Geometry check sheet. Reference: the model listing, model coordinates, mm. A direction names the side the tool comes from. Round coordinates to 2 decimals unless told otherwise and drop trailing zeros. Write each loop counter-clockwise with the first axis right and the second up, starting at its lowest first coordinate (ties: lowest second). Pieces come first, ordered by that corner, then holes.
Item 1: Cross-section at C-C (y = -19.05). Enter the section's corners in (x, z).
Item 2: Cross-section at B-B (x = 39.37). Enter the section's corners in (y, z).
Item 3: Access from +Z, -Z, +X, -X, +Y, -Y to the whole of each face (thin tool, end or side, straight path). Record for faces 1 (the face through (2, 25.38, 4)), 2 (the face through (42.481, -24, 4)), 3 (the face through (-26.433, -24, 4)).
Item 4: Scan lines: probe 1 along Y at (x, z) = (-3, 3.75); probe 2 along Y at (x, z) = (39.37, -0.65); probe 3 along Y at (x, z) = (-36.83, -1.2). Record each from-to range of solid material in increasing order.
Item 5: Cross-section at A-A (z = 4.25). Enter the section's corners in (x, y).
Item 6: Draft check along Y on faces 4 (the face through (-36.14, -25.46, -0.84)), 5 (the face through (2, 24, 8.34)), 6 (the face through (44, -20.35, 4)). Enter one of: pulls with the +Y half, pulls with the -Y half, needs draft (parallel to the pull), parting line crosses it, or undercut.
Item 7: Depth check by flat-ended pin: P1, Ø1, axis at x = -15, z = 1.5, coming from the -Y side; P2, Ø1.9, axis at y = 20, z = -0.5, coming from the +X side; P3, Ø3, axis at y = -24.5, z = 4, coming from the -X side; P4, Ø5, axis at x = 14, z = 1.5, coming from the -Y side. Enter the tip coordinate at first touch or a pass-through.
Item 8: Cross-section at D-D (y = -9). Enter the section's corners in (x, z), then the cut area to 3 significant figures.
Autodesk Fusion 360 part; units mm, degrees
sketch "Boceto1" plane through (0, 0, 0) normal (0, 0, 1) x (1, 0, 0)
  line L0 (-50.8, 26.67) -> (50.8, 26.67)
  line L1 (50.8, 26.67) -> (50.8, -26.67)
  line L2 (50.8, -26.67) -> (-50.8, -26.67)
  line L3 (-50.8, -26.67) -> (-50.8, 26.67)
  line L4 (-50.8, 0) -> (50.8, 0) construction
  circle A0 centre (-35.56, 24.13) radius 1.5
  circle A1 centre (39.37, 24.13) radius 1.5
  circle A2 centre (45.72, -24.13) radius 1.5
  circle A3 centre (-36.83, -24.13) radius 1.5
  circle A4 centre (15.24, -19.05) radius 1.5
  line L5 (45.2477, 26.67) -> (47.6517, 24.3349)
  line L6 (47.6517, 24.3349) -> (47.6517, 13.9338)
  line L7 (47.6517, 13.9338) -> (50.8, 10.0089)
  line L8 (47.6442, -26.67) -> (47.6442, -25.5537)
  line L9 (47.6442, -25.5537) -> (50.8, -23.002)
  line L10 (-32.1884, 25.38) -> (36.3857, 25.38)
  line L11 (36.3857, 25.38) -> (36.3857, 22.88)
  line L12 (36.3857, 22.88) -> (-32.1884, 22.88)
  line L13 (-32.1884, 22.88) -> (-32.1884, 25.38)
  line L14 (-32.1884, 25.38) -> (36.3857, 22.88) construction
  line L15 (36.3857, 25.38) -> (-32.1884, 22.88) construction
  line L16 (43.14, 24.13) -> (45.64, 24.13)
  line L17 (45.64, 24.13) -> (45.64, -20.35)
  line L18 (45.64, -20.35) -> (43.14, -20.35)
  line L19 (43.14, -20.35) -> (43.14, 24.13)
  line L20 (43.14, 24.13) -> (45.64, -20.35) construction
  line L21 (45.64, 24.13) -> (43.14, -20.35) construction
  line L22 (-26.4326, -22.88) -> (42.4806, -22.88)
  line L23 (42.4806, -22.88) -> (42.4806, -25.38)
  line L24 (42.4806, -25.38) -> (-26.4326, -25.38)
  line L25 (-26.4326, -25.38) -> (-26.4326, -22.88)
  line L26 (-26.4326, -22.88) -> (42.4806, -25.38) construction
  line L27 (42.4806, -22.88) -> (-26.4326, -25.38) construction
  point P0 (2.0986, 24.13)
  point P1 (44.39, 1.89)
  point P2 (8.024, -24.13)
  dimension "d2" = 53.34
  dimension "d3" = 101.6
  dimension "d4" = 13.97
  dimension "d5" = 15.24
  dimension "d7" = 2.54
  dimension "d8" = 50.8
  dimension "d9" = 96.52
  dimension "d10" = 90.17
  dimension "d11" = 7.62
  dimension "d12" = 66.04
  dimension "d13" = 3
  dimension "d17" = 2.5
  dimension "d18" = 2.5
  dimension "d19" = 2.5
extrude "Extruir1" add sketch "Boceto1" against normal blind 1.7 contours L0 L1 L2 L3 L5 L6 L7 L8 L9 | L10 L11 L12 L13 | L16 L17 L18 L19 | L22 L23 L24 L25
extrude "Extruir2" add sketch "Boceto1" along normal blind 8.34 contours L10 L11 L12 L13 | L16 L17 L18 L19 | L22 L23 L24 L25
Resolved:
1. outline: (-50.8, -1.7) - (13.74, -1.7) - (13.74, 0) - (-50.8, 0) - close; (16.74, -1.7) - (50.8, -1.7) - (50.8, 0) - (45.64, 0) - (45.64, 8.34) - (43.14, 8.34) - (43.14, 0) - (16.74, 0) - close
2. outline: (-26.67, -1.7) - (22.63, -1.7) - (22.63, 0) - (-22.88, 0) - (-22.88, 8.34) - (-25.38, 8.34) - (-25.38, 0) - (-26.67, 0) - close; (25.63, -1.7) - (26.67, -1.7) - (26.67, 0) - (25.63, 0) - close
3. face 1: +Z, +X, -X, +Y
3. face 2: +Z, +X, +Y, -Y
3. face 3: +Z, -X, -Y
4. probe 1: y = -25.38 to -22.88, 22.88 to 25.38
4. probe 2: y = -26.67 to 22.63, 25.63 to 26.67
4. probe 3: y = -26.67 to -25.63, -22.63 to 23.33, 24.93 to 26.67
5. outline: (-32.19, 22.88) - (36.39, 22.88) - (36.39, 25.38) - (-32.19, 25.38) - close; (-26.43, -25.38) - (42.48, -25.38) - (42.48, -22.88) - (-26.43, -22.88) - close; (43.14, -20.35) - (45.64, -20.35) - (45.64, 24.13) - (43.14, 24.13) - close
6. face 4: undercut
6. face 5: needs draft
6. face 6: pulls with the -Y half
7. P1: stops at y = -25.38
7. P2: stops at x = 47.65
7. P3: stops at x = -26.43
7. P4: stops at y = -26.67
8. outline: (-50.8, -1.7) - (50.8, -1.7) - (50.8, 0) - (45.64, 0) - (45.64, 8.34) - (43.14, 8.34) - (43.14, 0) - (-50.8, 0) - close
8. area: 194 mm2
